Design review of the part built by this model. Coordinates are the model's own, in mm. A direction names the side the tool comes from. Coordinates: 2 decimals unless noted, no trailing zeros. Order: outer loops, then holes, each group sorted by start corner. A loop starts at its lowest first (then second) coordinate and runs counter-clockwise, first axis right, second up. Notation, with made-up numbers: M 55.25,32.25 L 78.25,32.25 A21 ccw 78.25,54.25 Z; hole C 86,18.5 d2. An arc over 180 degrees is marked long. Answer in a Markdown table with one row per item.
Autodesk Inventor part; units mm, degrees
ref_plane "YZ Plane" through (0, 0, 0) normal (1, 0, 0) x (0, 1, 0)
ref_plane "XZ Plane" through (0, 0, 0) normal (0, 1, 0) x (-1, 0, 0)
ref_plane "XY Plane" through (0, 0, 0) normal (0, 0, 1) x (1, 0, 0)
sketch "Sketch1" plane through (0, 0, 0) normal (0, 0, 1) x (1, 0, 0)
  line L0 (-10, -16) -> (10, -16)
  line L1 (10, -16) -> (10, 16)
  line L2 (10, 16) -> (-10, 16)
  line L3 (-10, 16) -> (-10, -16)
  line L4 (-10, -16) -> (10, 16) construction
  line L5 (10, -16) -> (-10, 16) construction
  point P0 (0, 0)
  dimension "d0" = 32
  dimension "d1" = 20
extrude "Extrusion1" add sketch "Sketch1" along normal blind 3
sketch "Sketch2" plane through (0, 0, 0) normal (0, 0, -1) x (-1, 0, 0)
  line L0 (10, -16) -> (-10, -16)
  line L1 (-5.5, -16) -> (4.5, -16)
  line L2 (4.5, -16) -> (4.5, -19)
  line L3 (4.5, -19) -> (-5.5, -19)
  line L4 (-5.5, -19) -> (-5.5, -16)
  line L5 (-10, -16) -> (-10, 16)
  point P0 (0, 0)
  dimension "d4" = 10
  dimension "d5" = 3
  dimension "d6" = 4.5
extrude "Extrusion2" add sketch "Sketch2" against normal blind 3
sketch "Sketch3" plane through (0, 0, 0) normal (0, 0, -1) x (-1, 0, 0)
  line L0 (-10, -16) -> (-10, 16)
  line L1 (-10, -6) -> (-13, -6)
  line L2 (-13, -6) -> (-13, 4)
  line L3 (-13, 4) -> (-10, 4)
  line L4 (-10, 4) -> (-10, -6)
  line L5 (-5.5, -16) -> (-10, -16)
  point P0 (0, 0)
  dimension "d9" = 3
  dimension "d10" = 10
  dimension "d11" = 10
extrude "Extrusion3" add sketch "Sketch3" against normal blind 3
sketch "Sketch4" plane through (0, 0, 0) normal (0, 0, -1) x (-1, 0, 0)
  line L0 (10, 16) -> (10, -16)
  line L1 (10, -3.5) -> (0, -3.5)
  line L2 (0, -3.5) -> (0, -7)
  line L3 (0, -7) -> (10, -7)
  line L4 (10, -7) -> (10, -3.5)
  line L5 (10, -16) -> (4.5, -16)
  point P0 (0, 0)
  dimension "d14" = 10
  dimension "d15" = 3.5
  dimension "d16" = 9
extrude "Extrusion4" cut sketch "Sketch4" against normal blind 3
sketch "Sketch5" plane through (0, 0, 3) normal (0, 0, 1) x (1, 0, 0)
  line L0 (10, 16) -> (-10, 16)
  line L1 (5.5, 16) -> (-4.5, 16)
  line L2 (-4.5, 16) -> (-4.5, 19)
  line L3 (-4.5, 19) -> (5.5, 19)
  line L4 (5.5, 19) -> (5.5, 16)
  line L5 (5.5, -19) -> (5.5, -16)
  point P0 (0, 0)
  dimension "d19" = 10
  dimension "d20" = 3
extrude "Extrusion5" add sketch "Sketch5" against normal blind 3
properties part number "Board holders"
(1) Add section C-C, the plane y = -6.5. Give the boundary of the cut face in (x, z).
Return value:
| item | result |
|---|---|
| outline | M 0,0 L 10,0 L 10,3 L 0,3 Z |
(2) Add section B-B, the plane z = 0.65. Give the boundary of the cut face in (x, y), and give its area (3 significant figures).
Return value:
| item | result |
|---|---|
| outline | M -10,-16 L -4.5,-16 L -4.5,-19 L 5.5,-19 L 5.5,-16 L 10,-16 L 10,-6 L 13,-6 L 13,4 L 10,4 L 10,16 L 5.5,16 L 5.5,19 L -4.5,19 L -4.5,16 L -10,16 L -10,-3.5 L 0,-3.5 L 0,-7 L -10,-7 Z |
| area | 695 mm2 |
(3) Insertion check: pin 1 Ø1.5 at (y, z) = (-17, 2) entering from -X; pin 2 Ø0.9 at (x, z) = (9, 1) entering from +Y; pin 3 Ø1.5 at (y, z) = (17.5, 1.5) entering from +X. Each pin has a flat end and moves straight along its axis. Give the tip position at first contact, or say it passes through.
Return value:
| item | result |
|---|---|
| pin 1 | stops at x = -4.5 |
| pin 2 | stops at y = 16 |
| pin 3 | stops at x = 5.5 |
(4) Add section D-D, the plane x = -1.5. Give the boundary of the cut face in (y, z), and give its area (4 significant figures).
Return value:
| item | result |
|---|---|
| outline | M -19,0 L -7,0 L -7,3 L -19,3 Z; M -3.5,0 L 19,0 L 19,3 L -3.5,3 Z |
| area | 103.5 mm2 |
(5) For faces 1 (the flat face through (-5, -3.5, 1)), 2 (the flat face through (11, -6, 1)), 3 (the flat face through (-4.5, -17, 1)), list the 3-axis set-ups (+Z, -Z, +X, -X, +Y, -Y) from which the entire face can be reached by the end or side of a thin tool; tool diameter is ignored.
Return value:
| item | result |
|---|---|
| face 1 | +Z, -Z, -X |
| face 2 | +Z, -Z, +X, -Y |
| face 3 | +Z, -Z, -X, -Y |
(6) For line 1 along Y through (x, z) = (-7.5, 1.3); line 2 along Y through (x, z) = (-1, 1.6); line 3 along X through (y, z) = (9.5, 1.55), list the stretches that pass through material, from the lowest coordinate up. Write a range as from..to.
Return value:
| item | result |
|---|---|
| line 1 | y = -16..-7, -3.5..16 |
| line 2 | y = -19..-7, -3.5..19 |
| line 3 | x = -10..10 |
(7) Add section A-A, the plane x = -7.5. Give the boundary of the cut face in (y, z), and give its area (3 significant figures).
Return value:
| item | result |
|---|---|
| outline | M -16,0 L -7,0 L -7,3 L -16,3 Z; M -3.5,0 L 16,0 L 16,3 L -3.5,3 Z |
| area | 85.5 mm2 |
